Source: CAD feature listing. Evaluate the final solid. Frame: model axes, mm. A direction names the side the tool comes from. Coordinates: 2 decimals unless noted, no trailing zeros. Loops run counter-clockwise (first coordinate to the right, second up) from the corner with the lowest first, then second, coordinate; pieces in that order, holes last.
Item 1: Reachability of faces 1 (the cylindrical face through (0.631, 23.743, 2.003)), 2 (the flat face through (0, 3.828, 0)) from +Z, -Z, +X, -X, +Y, -Y: full face, straight path, thin tool, end or side. Return the list, or none.
Item 2: Section query B-B, the plane x = 0. Return the cut outline in (y, z), then the cut area to 3 significant figures.
Item 3: Section query C-C, the plane y = 24.25. Return the cut outline in (x, z), then the cut area to 3 significant figures.
Item 4: Line query: probe 1 along Y at (x, z) = (5.75, 4.5); probe 2 along X at (y, z) = (12.25, 6.75); probe 3 along Z at (x, y) = (-1, 22.5). Output: solid intervals per line, ascending.
Item 5: Section query A-A, the plane z = 0. Return the cut outline in (x, y).
Item 6: Section query D-D, the plane z = 4.25. Return the cut outline in (x, y), then the cut area to 4 significant figures.
```python
from build123d import *

# Parameters (mm, degrees)
SKETCH1_R           = 6
BOSS_EXTRUDE1_DEPTH = 25
SKETCH2_R           = 3
BOSS_EXTRUDE2_DEPTH = 7
SCALE1_SCALE        = 0.7


with BuildPart() as part:
    # Sketch1 → Boss-Extrude1 (new body)
    # profile 1 of 2: a face of its own
    with BuildSketch(Plane(origin=(0, 0, 0), x_dir=(1, 0, 0), z_dir=(0, 1, 0))):
        with BuildLine():
            ThreePointArc((-11, 9), (-10.414213562, 10.414213562), (-9, 11))
            Line((-9, 11), (9, 11))
            ThreePointArc((9, 11), (10.414213562, 10.414213562), (11, 9))
            Line((11, 9), (11, -9))
            ThreePointArc((11, -9), (10.414213562, -10.414213562), (9, -11))
            Line((9, -11), (-9, -11))
            ThreePointArc((-9, -11), (-10.414213562, -10.414213562), (-11, -9))
            Line((-11, -9), (-11, 9))
        make_face()
        Circle(SKETCH1_R, mode=Mode.SUBTRACT)
    # profile 2 of 2: a face of its own
    with BuildSketch(Plane(origin=(0, 0, 0), x_dir=(1, 0, 0), z_dir=(0, 1, 0))):
        Circle(SKETCH1_R)
    extrude(amount=BOSS_EXTRUDE1_DEPTH)

    # Sketch2 → Boss-Extrude2 (add)
    with BuildSketch(Plane(origin=(0, 25, 0), x_dir=(1, 0, 0), z_dir=(0, 1, 0))):
        with Locations(Location((0, 0, 0), (0, 0, 270))):
            Circle(SKETCH2_R)
    extrude(amount=BOSS_EXTRUDE2_DEPTH)


with BuildPart() as part_1:
    # Scale1: scaled about (0, 12.759310903, 0)
    add(part.part.scale(SCALE1_SCALE).moved(Location((0, 3.827793271, 0))))


solid = part_1.part
```
Verdict:
1. face 1: +Y
1. face 2: +Z, -Z, +X, -X, -Y
2. outline: (3.83, -7.7) - (21.33, -7.7) - (21.33, -2.1) - (26.23, -2.1) - (26.23, 2.1) - (21.33, 2.1) - (21.33, 7.7) - (3.83, 7.7) - close
2. area: 290 mm2
3. outline: circle Ø4.2 at (0, 0)
3. area: 13.9 mm2
4. probe 1: y = 3.83 to 21.33
4. probe 2: x = -7.63 to 7.63
4. probe 3: z = -1.85 to 1.85
5. outline: (-7.7, 3.83) - (7.7, 3.83) - (7.7, 21.33) - (2.1, 21.33) - (2.1, 26.23) - (-2.1, 26.23) - (-2.1, 21.33) - (-7.7, 21.33) - close
6. outline: (-7.7, 3.83) - (7.7, 3.83) - (7.7, 21.33) - (-7.7, 21.33) - close
6. area: 269.5 mm2
